Here's how the part is built. I have some questions about the finished solid (model axes, mm). Face numbers are marked on the shaded views. A direction names the side the tool comes from. Give positions to 0.01 mm unless a question says otherwise; leave off trailing zeros. Order: outer loops, then holes, each group sorted by start corner. A loop starts at its lowest first (then second) coordinate and runs counter-clockwise, first axis right, second up. Notation, with made-up numbers: (-16, 68) -> (-10, 68) arc R6 ccw to (-10, 72) -> close; hole circle Ø10 at (6, 41). An arc over 180 degrees is marked (long way). Write each question's results on one line, items separated by ' | '. Start each with the question number.
Q1. Imagine slicing it at D-D, the plane x = 8.5. State how many separate pieces and enclosed holes the cut face has, then the cut area to 3 significant figures.
Q2. Imagine slicing it at C-C, the plane x = -12. Please give me the cut outline in (y, z).
Q3. Imagine slicing it at A-A, the plane x = -5. Please give me the cut outline in (y, z).
Q4. Imagine slicing it at B-B, the plane z = -3. Please give me the cut outline in (x, y).
Q5. I need wall thicknesses on line 1 along Y through (x, z) = (-5, -6.25); line 2 along Y through (x, z) = (11.25, -3.5); line 3 along Y through (x, z) = (11.75, 2). Which ranges of each line are inside material? Lowest first, please. Write a range as [from, to].
Q6. I'm going to push flat-ended pins straight in: pin 1 (3.5 mm diameter, centred on x = -0.5, z = -4.5, fed in from -Y); pin 2 (5 mm diameter, centred on x = 3, z = 11, fed in from -Y); pin 3 (8.5 mm diameter, centred on x = 0, y = 36.5, fed in from +Z). Where does each tip first touch, or does it pass through?
Q7. Thinking about a two-plate mould opening in Y: for the marked faces 1, 2 and 3, which applies, pulls with the +Y half, pulls with the -Y half, needs draft (parallel to the pull), parting line crosses it, or undercut?
Q8. For the marked faces 4, 5 and 6, which set-ups out of +Z, -Z, +X, -X, +Y, -Y let a thin tool reach every point of the face, with its end or its side?
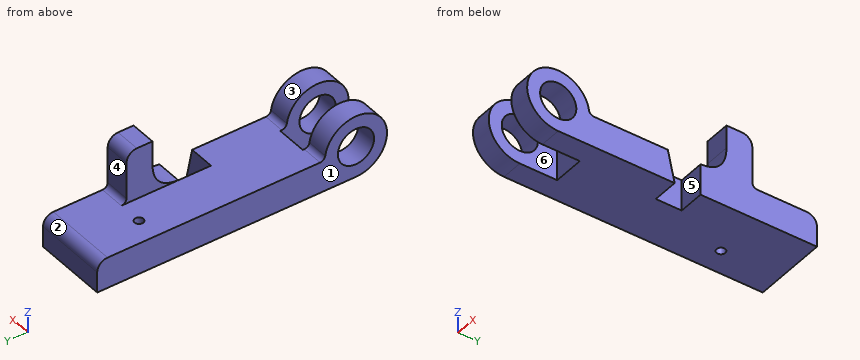
```python
from build123d import *

# Parameters (mm, degrees)
F0_R         = 7
F1_DEPTH     = 14.4
F2_W         = 12
F2_H         = 26.4532811218
F2_H_2       = 2.4532811218
F3_DEPTH     = 15
F4_R         = 2
F6_DEPTH     = 25
F7_W         = 18.8
F7_H         = 33.2335345083
F7_H_2       = 13.5664814711
F8_DEPTH     = 25
F11_DEPTH    = 10
F12_T4_DEPTH = 10


# Not quite as in the source:
# - a fillet or chamfer that OpenCascade refuses, or shapes differently, is made with other operations: its cross-section is extruded or revolved along the edge and cut away or added


with BuildPart() as f1:
    # F0 (on Right) → F1 (new body, symmetric)
    with BuildSketch(Plane.YZ):
        with BuildLine():
            Line((42.36, 0), (12, 0))
            ThreePointArc((12, 0), (-8.4852813742, 8.4852813742), (0, -12))
            Line((0, -12), (47.36, -12))
            Line((47.36, -12), (42.36, 0))
        make_face()
        Circle(F0_R, mode=Mode.SUBTRACT)
        Polygon((57.36, 0), (42.36, 0), (47.36, -12), (57.36, -12), align=None)
        with BuildLine():
            Line((65, 0), (57.36, 0))
            Line((57.36, 0), (57.36, -12))
            Line((57.36, -12), (100, -12))
            Line((100, -12), (100, -4))
            ThreePointArc((100, -4), (98.8284271247, -1.1715728753), (96, 0))
            Line((96, 0), (77, 0))
            ThreePointArc((77, 0), (75.5857864376, 0.5857864376), (75, 2))
            Line((75, 2), (75, 16))
            ThreePointArc((75, 16), (73.8284271247, 18.8284271247), (71, 20))
            Line((71, 20), (65, 20))
            Line((65, 20), (65, 0))
        make_face()
    extrude(amount=F1_DEPTH, both=True)

    # F2 (on face) → F3 (cut, symmetric)
    with BuildSketch(Plane.XY):
        with Locations((0, -1.2266405609)):
            Rectangle(F2_W, F2_H)
        with Locations((0, 13.2266405609)):
            Rectangle(F2_W, F2_H_2)
    extrude(amount=F3_DEPTH, both=True, mode=Mode.SUBTRACT)

    # F4
    f4_edges = [f1.edges().sort_by_distance(p)[0] for p in [
        (10.2, 12, 0),
        (-10.2, 12, 0),
    ]]
    fillet(f4_edges, radius=F4_R)

    # F5 (on face) → F6 (cut)
    with BuildSketch(Plane.XY):
        with BuildLine():
            Line((-5, 77), (-6.7, 77))
            ThreePointArc((-6.7, 77), (-5, 75.3), (-3.3, 77))
            Line((-3.3, 77), (-5, 77))
        make_face()
        with BuildLine():
            ThreePointArc((-3.3, 77), (-5, 78.7), (-6.7, 77))
            Line((-6.7, 77), (-5, 77))
            Line((-5, 77), (-3.3, 77))
        make_face()
    extrude(amount=-F6_DEPTH, mode=Mode.SUBTRACT)

    # F7 (on face) → F8 (cut)
    with BuildSketch(Plane.XY):
        with Locations((-5, 81.6167672542)):
            Rectangle(F7_W, F7_H)
        with Locations((-5, 58.2167592645)):
            Rectangle(F7_W, F7_H_2)
    extrude(amount=F8_DEPTH, mode=Mode.SUBTRACT)

    # F10 (on face) → F11 (cut)
    with BuildSketch(Plane.YZ.offset(14.4)):
        Polygon((55, -12), (55, 0), (42.36, 0), (45, -12), align=None)
    extrude(amount=-F11_DEPTH, mode=Mode.SUBTRACT)

    # F12: fillet of radius 11.1053823869 on 1 edges, made by hand


with BuildPart() as f12_tool2:
    # F12_s3 → F12_t4 (new body)
    with BuildSketch(Plane.YZ.offset(14.4)):
        with BuildLine():
            add(Edge.make_bspline(
                [(53.8946176131, 0), (65, 0), (65, 11.1053823869)],
                knots=[0, 0, 0, 1, 1, 1], degree=2, weights=[1, 1, 1]))
            Line((65, 11.1053823869), (65, 0))
            Line((65, 0), (53.8946176131, 0))
        make_face()
    extrude(amount=-F12_T4_DEPTH)

    split(bisect_by=Plane.XZ.offset(-55), keep=Keep.BOTTOM)


with BuildPart() as f1_1:
    add(f1.part)

    # F12_t1: union F12_tool2
    add(f12_tool2.part)


solid = f1_1.part
```
Geometry check:
1) separate pieces: 2 | enclosed holes: 1 | area: 1,460 mm²
2) outline: (0, -12) -> (100, -12) -> (100, -4) arc R4 ccw to (96, 0) -> (13.86, 0) arc R2 cw to (11.88, 1.71) arc R12 ccw (long way) to start; hole circle Ø14 at (0, 0)
3) outline: (14.45, -12) -> (75.3, -12) -> (75.3, 0) -> (14.45, 0) -> close; (78.7, -12) -> (100, -12) -> (100, -4) arc R4 ccw to (96, 0) -> (78.7, 0) -> close
4) outline: (-14.4, -11.62) -> (-6, -11.62) -> (-6, -6.32) -> (-14.4, -6.32) -> close; (-14.4, 6.32) -> (-6, 6.32) -> (-6, 14.45) -> (6, 14.45) -> (6, 6.32) -> (14.4, 6.32) -> (14.4, 43.02) -> (4.4, 43.02) -> (4.4, 55) -> (14.4, 55) -> (14.4, 99.87) -> (-14.4, 99.87) -> close; (6, -11.62) -> (14.4, -11.62) -> (14.4, -6.32) -> (6, -6.32) -> close; hole circle Ø3.4 at (-5, 77)
5) line 1: [14.45, 75.3], [78.7, 100] | line 2: [-11.48, -6.06], [6.06, 43.13], [55, 99.97] | line 3: [-11.83, -6.71], [6.71, 11.83], [61.32, 75]
6) pin 1: y = 14.45 | pin 2: y = 64.88 | pin 3: z = 0
7) face 1: needs draft | face 2: pulls with the +Y half | face 3: undercut
8) face 4: +Z, +X, -X, +Y | face 5: +Z, -Z, +X | face 6: +Z, -Z, -Y
